```python
from build123d import *

# Parameters (mm, degrees)
BOX_W        = 30
BOX_H        = 30
BOX_DEPTH    = 10
BOX001_W     = 26
BOX001_H     = 26
BOX001_DEPTH = 8
SKETCH_R     = 2
PAD_DEPTH    = 2


with BuildPart() as part:
    # Box → Box (join)
    with BuildSketch(Plane.XY):
        with Locations((15, 15)):
            Rectangle(BOX_W, BOX_H)
    extrude(amount=BOX_DEPTH)

    # Box001 → Box001 (cut)
    with BuildSketch(Plane(origin=(2, 2, 2), x_dir=(1, 0, 0), z_dir=(0, 0, 1))):
        with Locations((13, 13)):
            Rectangle(BOX001_W, BOX001_H)
    extrude(amount=BOX001_DEPTH, mode=Mode.SUBTRACT)

    # Sketch → Pad (join)
    with BuildSketch(Plane.XY):
        with BuildLine():
            Line((0, 35), (0, 30))
            ThreePointArc((0, 30), (1.464466, 26.464466), (5, 25))
            Line((5, 25), (25, 25))
            ThreePointArc((25, 25), (28.535534, 26.464466), (30, 30))
            Line((30, 30), (30, 35))
            ThreePointArc((30, 35), (28.535534, 38.535534), (25, 40))
            Line((25, 40), (5, 40))
            ThreePointArc((5, 40), (1.464466, 38.535534), (0, 35))
        make_face()
        with Locations((5, 35)):
            Circle(SKETCH_R, mode=Mode.SUBTRACT)
        with Locations((25, 35)):
            Circle(SKETCH_R, mode=Mode.SUBTRACT)
    extrude(amount=PAD_DEPTH)


solid = part.part
```
Verification items for the finished model (mm, model axes). A direction names the side the tool comes from. Round coordinates to 2 decimals unless told otherwise and drop trailing zeros. Write each loop counter-clockwise with the first axis right and the second up, starting at its lowest first coordinate (ties: lowest second). Pieces come first, ordered by that corner, then holes.
1. Scan lines: L1, parallel to Y at x = 15.5, z = 5.75; L2, parallel to Y at x = 5, z = 1.45. Record each from-to range of solid material in increasing order.
2. Section check A-A on z = 2.75. Enter the section's corners in (x, y).
3. Gauge pin test, flat ends, axial feed: P1, Ø3, axis at x = 4, y = 8, coming from the +Z side; P2, Ø2.5, axis at x = 12.5, z = 5.5, coming from the +Y side; P3, Ø3.5, axis at x = 5, y = 35, coming from the +Z side. Record the tip position at first contact, or that the pin passes through.
4. Access from +Z, -Z, +X, -X, +Y, -Y to the whole of each face (thin tool, end or side, straight path). Record for faces 1 (the flat face through (28, 15, 6)), 2 (the flat face through (15, 35, 2)), 3 (the flat face through (15, 0, 5)).
5. Section check D-D on x = 12. Enter the section's corners in (y, z).
6. Draft check along X on faces 4 (the flat face through (15, 2, 6)), 5 (the flat face through (30, 17, 5)), 6 (the flat face through (1, 15, 10)). Enter one of: +X half, -X half, draft (parallel to the pull), parting line (faces both ways), or undercut.
7. Section check B-B on x = 6. Enter the section's corners in (y, z), plus the area to 3 significant figures.
8. Section check C-C on y = 34. Enter the section's corners in (x, z), plus the area to 3 significant figures.
Answer:
1. L1: y = 0 to 2, 28 to 30
1. L2: y = 0 to 33, 37 to 40
2. outline: (0, 0) - (30, 0) - (30, 30) - (0, 30) - close; hole (2, 2) - (28, 2) - (28, 28) - (2, 28) - close
3. P1: stops at z = 2
3. P2: stops at y = 30
3. P3: passes through
4. face 1: +Z
4. face 2: +Z, +X, -X, +Y
4. face 3: +Z, -Z, +X, -X, -Y
5. outline: (0, 0) - (40, 0) - (40, 2) - (30, 2) - (30, 10) - (28, 10) - (28, 2) - (2, 2) - (2, 10) - (0, 10) - close
6. face 4: undercut
6. face 5: +X half
6. face 6: draft
7. outline: (0, 0) - (33.27, 0) - (33.27, 2) - (30, 2) - (30, 10) - (28, 10) - (28, 2) - (2, 2) - (2, 10) - (0, 10) - close; (36.73, 0) - (40, 0) - (40, 2) - (36.73, 2) - close
7. area: 105 mm2
8. outline: (0, 0) - (3.27, 0) - (3.27, 2) - (0, 2) - close; (6.73, 0) - (23.27, 0) - (23.27, 2) - (6.73, 2) - close; (26.73, 0) - (30, 0) - (30, 2) - (26.73, 2) - close
8. area: 46.1 mm2
